from build123d import *

# Parameters (mm, degrees)
SKETCH001_R        = 2.963423
POCKET_DEPTH       = 233.757944
POLARPATTERN_COUNT = 6
POCKET001_DEPTH    = 41
CHAMFER_SIZE       = 2


with BuildPart() as part:
    # Sketch → Revolution (revolve)
    with BuildSketch(Plane.XZ):
        Polygon((-30, 48.502502), (-30, 23.544098), (-16.870987, 23.544098), (-16.870987, -20.881861), (-30, -20.881861), (-30, -27.204653), (0, -27.204653), (0, 48.502502), align=None)
    revolve(axis=Axis((0, 0, 0), (0, 0, 1)))

    # Sketch001 (on Face4 of Revolution) → Pocket (cut, through all)
    with BuildSketch(Plane(origin=(0, 0, -20.881861), x_dir=(-1, 0, 0), z_dir=(0, 0, 1))):
        with Locations((0, -24.60987)):
            Circle(SKETCH001_R)
    pocket = extrude(amount=-POCKET_DEPTH, mode=Mode.SUBTRACT)

    # PolarPattern: Pocket ×6 about axis
    polarpattern_axis = Axis((0, 0, -20.881861), (0, 0, 1))
    for i in range(1, POLARPATTERN_COUNT):
        add(pocket.rotate(polarpattern_axis, i * 360 / POLARPATTERN_COUNT), mode=Mode.SUBTRACT)

    # Sketch002 → Pocket001 (cut, symmetric)
    with BuildSketch(Plane.YZ):
        Polygon((-46.942223, 56.337571), (-46.942223, 49.89431), (-46.942223, -10.657207), (-18.07431, -10.657207), (-11.208346, 49.89431), (-6.428893, 49.89431), (-6.428893, 33.567371), (6.428893, 33.567371), (6.428893, 49.89431), (11.208346, 49.89431), (18.07431, -10.657207), (46.942223, -10.657207), (46.942223, 49.89431), (46.942223, 56.337571), align=None)
    extrude(amount=POCKET001_DEPTH, both=True, mode=Mode.SUBTRACT)

    # Chamfer
    chamfer_edges = [part.edges().sort_by_distance(p)[0] for p in [
        (0, -6.428893, 33.567371),
        (0, 6.428893, 33.567371),
    ]]
    chamfer(chamfer_edges, length=CHAMFER_SIZE)


solid = part.part
Read the model definition and answer for the solid it produces. Units are mm, in the model's axes. A direction names the side the tool comes from. Round coordinates to 2 decimals unless told otherwise and drop trailing zeros. Order: outer loops, then holes, each group sorted by start corner. A loop starts at its lowest first (then second) coordinate and runs counter-clockwise, first axis right, second up.
1) The part is cut by section D-D on x = -21.5. Write down the section's boundary in (y, z), plus the area to 3 significant figures.
2) Flat-ended cylindrical pins translate along their axes: pin 1 (6.5 mm diameter, centred on x = -4.5, z = 41.5, fed in from -Y); pin 2 (1.5 mm diameter, centred on x = 18.5, y = 24, fed in from +Z); pin 3 (5 mm diameter, centred on x = -7, z = -1.5, fed in from +Y); pin 4 (7 mm diameter, centred on x = -21.31, y = -12.3, fed in from -Z). Find the tip coordinate at first contact, or state that the pin passes through.
3) The mould has two halves that part along Y. Classify faces 1 (the face through (0.39, 13.47, 29.96)), 2 (the face through (30, 0, 33)), 3 (the face through (-24.05, -11.17, -24)), 4 (the face through (13, 13, -20.882)): released by +Y, released by -Y, zero draft, split by the parting line, or undercut.
4) The part is cut by section A-A on x = 0. Write down the section's boundary in (y, z) (1 decimal), plus the area to 3 significant figures.
5) Straight lines are drawn through the part: L1, parallel to Y at x = 0, z = -22.75; L2, parallel to Z at x = -21.5, y = -8.5; L3, parallel to Z at x = -26, y = -2.5. For each, find the intervals that lie inside material, in ascending order.
6) The part is cut by section B-B on z = 42. Write down the section's boundary in (x, y), plus the area to 3 significant figures.
7) For faces 5 (the face through (23.497, -14.308, -23.999)), 6 (the face through (-9.07, -14.226, 1.02)), 7 (the face through (0, -6.429, 42)), 8 (the face through (0, 0, -27.205)), determine the directions among +Z, -Z, +X, -X, +Y, -Y from which every point of the face is accessible in a straight line to the end or side of a thin tool.
8) The part is cut by section C-C on y = 0. Write down the section's boundary in (x, z), plus the area to 3 significant figures.
Resolved:
1. outline: (-20.92, -27.2) - (-15.26, -27.2) - (-15.26, -20.88) - (-20.92, -20.88) - close; (-14.2, 23.54) - (14.2, 23.54) - (11.37, 48.5) - (6.43, 48.5) - (6.43, 35.57) - (4.43, 33.57) - (-4.43, 33.57) - (-6.43, 35.57) - (-6.43, 48.5) - (-11.37, 48.5) - close; (-9.35, -27.2) - (9.35, -27.2) - (9.35, -20.88) - (-9.35, -20.88) - close; (15.26, -27.2) - (20.92, -27.2) - (20.92, -20.88) - (15.26, -20.88) - close
1. area: 640 mm2
2. pin 1: stops at y = -12.53
2. pin 2: stops at z = -20.88
2. pin 3: stops at y = 16.26
2. pin 4: stops at z = -27.2
3. face 1: released by +Y
3. face 2: split by the parting line
3. face 3: undercut
3. face 4: zero draft
4. outline: (-30, -27.2) - (-27.6, -27.2) - (-27.6, -20.9) - (-30, -20.9) - close; (-21.6, -27.2) - (21.6, -27.2) - (21.6, -20.9) - (16.9, -20.9) - (16.9, 0) - (11.4, 48.5) - (6.4, 48.5) - (6.4, 35.6) - (4.4, 33.6) - (-4.4, 33.6) - (-6.4, 35.6) - (-6.4, 48.5) - (-11.4, 48.5) - (-16.9, 0) - (-16.9, -20.9) - (-21.6, -20.9) - close; (27.6, -27.2) - (30, -27.2) - (30, -20.9) - (27.6, -20.9) - close
4. area: 2,190 mm2
5. L1: y = -30 to -27.57, -21.65 to 21.65, 27.57 to 30
5. L2: z = -27.2 to -20.88, 23.54 to 48.5
5. L3: z = -27.2 to -20.88, 23.54 to 33.57
6. outline: (-29.3, -6.43) arc R30 ccw to (-27.45, -12.1) - (27.45, -12.1) arc R30 ccw to (29.3, -6.43) - close; (-29.3, 6.43) - (29.3, 6.43) arc R30 ccw to (27.45, 12.1) - (-27.45, 12.1) arc R30 ccw to start
6. area: 646 mm2
7. face 5: -Z
7. face 6: none
7. face 7: +Z, +X, -X
7. face 8: -Z, +X, -X, +Y, -Y
8. outline: (-30, -27.2) - (30, -27.2) - (30, -20.88) - (16.87, -20.88) - (16.87, 23.54) - (30, 23.54) - (30, 33.57) - (-30, 33.57) - (-30, 23.54) - (-16.87, 23.54) - (-16.87, -20.88) - (-30, -20.88) - close
8. area: 2,480 mm2
